from build123d import *

# Parameters (mm, degrees)
SKETCH1_R           = 20.32
SKETCH1_R_2         = 3.175
SKETCH1_R_3         = 6.35
BOSS_EXTRUDE1_DEPTH = 12.7
SKETCH2_R           = 3.175
CUT_EXTRUDE1_DEPTH  = 21.32


with BuildPart() as part:
    # Sketch1 → Boss-Extrude1 (new body)
    with BuildSketch(Plane.XY):
        Circle(SKETCH1_R)
        with Locations((-9.525, -9.525)):
            Circle(SKETCH1_R_2, mode=Mode.SUBTRACT)
        with Locations((9.525, -9.525)):
            Circle(SKETCH1_R_2, mode=Mode.SUBTRACT)
        with Locations((9.525, 9.525)):
            Circle(SKETCH1_R_2, mode=Mode.SUBTRACT)
        with Locations((-9.525, 9.525)):
            Circle(SKETCH1_R_2, mode=Mode.SUBTRACT)
        Circle(SKETCH1_R_3, mode=Mode.SUBTRACT)
    extrude(amount=BOSS_EXTRUDE1_DEPTH)

    # Sketch2 → Cut-Extrude1 (cut, through all)
    with BuildSketch(Plane(origin=(0, 0, 0), x_dir=(0, 0, -1), z_dir=(1, 0, 0))):
        with Locations((-6.35, 0)):
            Circle(SKETCH2_R)
    extrude(amount=-CUT_EXTRUDE1_DEPTH, mode=Mode.SUBTRACT)


solid = part.part
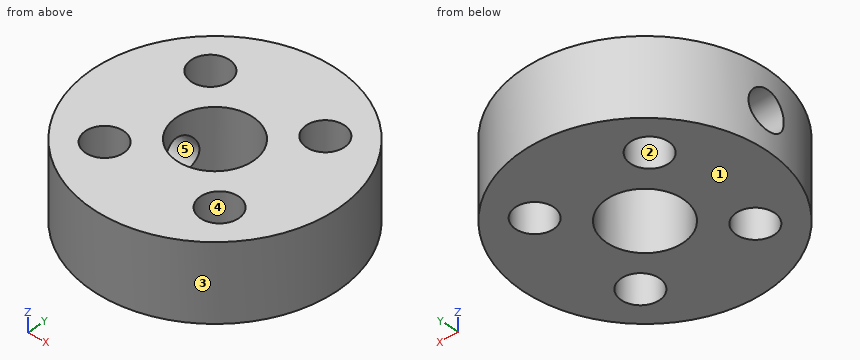
Input: part model. Units: mm. Frame: model coordinates. Face numbers are marked on the shaded views. A direction names the side the tool comes from. Coordinates: 2 decimals unless noted, no trailing zeros. Loops run counter-clockwise (first coordinate to the right, second up) from the corner with the lowest first, then second, coordinate; pieces in that order, holes last.
(1) Section D-D on x = -11. Return the cut outline in (y, z) (3 decimals), then the cut area to 3 significant figures.
(2) First-contact query: pin 1 Ø2 at (x, z) = (2, 2) entering from -Y; pin 2 Ø5 at (x, y) = (9.525, 9.525) entering from +Z; pin 3 Ø4 at (y, z) = (3, 8) entering from -X; pin 4 Ø2 at (x, y) = (-6.5, -15.5) entering from -Z. Flat tips, straight axial feed; report the tip coordinate or a pass-through.
(3) Material intervals for probe 1 along Y at (x, z) = (8, 1.25); probe 2 along Y at (x, z) = (-11, 5.5); probe 3 along Y at (x, z) = (0, 1.5), sorted ascending.
(4) Pull-direction query (Y, two-part tool) for the marked faces 1, 2 and 3; classes: released by +Y, released by -Y, zero draft, split by the parting line, or undercut.
(5) Section C-C on z = 6. Return the cut outline in (x, y) (3 decimals).
(6) Section B-B on x = 0. Return the cut outline in (y, z).
(7) Section A-A on y = 0. Return the cut outline in (x, z) (3 decimals), then the cut area to 3 significant figures.
(8) Set-up query: the marked faces 4 and 5. Return all of +Z, -Z, +X, -X, +Y, -Y with unobstructed straight access to the full face (end or side cutting, diameter ignored); none if empty.
Data:
1. outline: (-17.085, 0) - (-12.337, 0) - (-12.337, 12.7) - (-17.085, 12.7) - close; (-6.713, 0) - (6.713, 0) - (6.713, 12.7) - (-6.713, 12.7) - close; (12.337, 0) - (17.085, 0) - (17.085, 12.7) - (12.337, 12.7) - close; hole circle Ø6.35 at (0, 6.35)
1. area: 259 mm2
2. pin 1: stops at y = -20.3
2. pin 2: passes through
2. pin 3: stops at x = -20.27
2. pin 4: stops at z = 0
3. probe 1: y = -18.68 to -12.31, -6.74 to 6.74, 12.31 to 18.68
3. probe 2: y = -17.09 to -12.34, -6.71 to -3.06, 3.06 to 6.71, 12.34 to 17.09
3. probe 3: y = -20.32 to -6.35, 6.35 to 20.32
4. face 1: zero draft
4. face 2: undercut
4. face 3: split by the parting line
5. outline: (-20.073, -3.156) arc R20.32 ccw (long way) to (-20.073, 3.156) - (-5.51, 3.156) arc R6.35 cw (long way) to (-5.51, -3.156) - close; hole circle Ø6.35 at (-9.525, -9.525); hole circle Ø6.35 at (-9.525, 9.525); hole circle Ø6.35 at (9.525, -9.525); hole circle Ø6.35 at (9.525, 9.525)
6. outline: (-20.32, 0) - (-6.35, 0) - (-6.35, 12.7) - (-20.32, 12.7) - close; (6.35, 0) - (20.32, 0) - (20.32, 12.7) - (6.35, 12.7) - close
7. outline: (-20.32, 0) - (-6.35, 0) - (-6.35, 3.175) - (-20.32, 3.175) - close; (-20.32, 9.525) - (-6.35, 9.525) - (-6.35, 12.7) - (-20.32, 12.7) - close; (6.35, 0) - (20.32, 0) - (20.32, 12.7) - (6.35, 12.7) - close
7. area: 266 mm2
8. face 4: +Z, -Z
8. face 5: -X
